The model under review builds one solid part; all positions refer to its coordinate system, in mm. A direction names the side the tool comes from. Coordinates: 2 decimals unless noted, no trailing zeros. Write each loop counter-clockwise with the first axis right and the second up, starting at its lowest first coordinate (ties: lowest second). Pieces come first, ordered by that corner, then holes. Notation, with made-up numbers: (70, -25.5) - (100, -25.5) arc R19 cw to (100, -10.5) - close; hole circle Ø4 at (60.25, 59). An arc over 180 degrees is marked (long way). Answer as CSV lines item,"result". Start each with the question number.
```python
from build123d import *

# Parameters (mm, degrees)
BOSS_EXTRUDE1_DEPTH = 8
CUT_EXTRUDE4_DEPTH  = 1.7
CUT_EXTRUDE5_DEPTH  = 7.4
CUT_EXTRUDE6_DEPTH  = 4.5
SKETCH3_R           = 2.2
CUT_EXTRUDE7_DEPTH  = 6
SKETCH1_10_R        = 1.6
CUT_EXTRUDE8_DEPTH  = 60.512855754


with BuildPart() as part:
    # Sketch1 → Boss-Extrude1 (new body)
    with BuildSketch(Plane.XY):
        with BuildLine():
            ThreePointArc((-32.17302157, 26.528978176), (-41.7, 0), (-32.17302157, -26.528978176))
            ThreePointArc((-32.17302157, -26.528978176), (-31.395541085, -31.395541085), (-26.528978176, -32.17302157))
            ThreePointArc((-26.528978176, -32.17302157), (0, -41.7), (26.528978176, -32.17302157))
            ThreePointArc((26.528978176, -32.17302157), (31.395541085, -31.395541085), (32.17302157, -26.528978176))
            ThreePointArc((32.17302157, -26.528978176), (41.7, 0), (32.17302157, 26.528978176))
            ThreePointArc((32.17302157, 26.528978176), (31.395541085, 31.395541085), (26.528978176, 32.17302157))
            ThreePointArc((26.528978176, 32.17302157), (0, 41.7), (-26.528978176, 32.17302157))
            ThreePointArc((-26.528978176, 32.17302157), (-31.395541085, 31.395541085), (-32.17302157, 26.528978176))
        make_face()
    extrude(amount=BOSS_EXTRUDE1_DEPTH)

    # Sketch1_7 → Cut-Extrude4 (cut)
    with BuildSketch(Plane.XY):
        with BuildLine():
            Line((-4.282842712, 9.374011537), (-9.475230868, 14.566399692))
            ThreePointArc((-9.475230868, 14.566399692), (-14.566399692, 14.566399692), (-14.566399692, 9.475230868))
            Line((-14.566399692, 9.475230868), (-9.374011537, 4.282842712))
            ThreePointArc((-9.374011537, 4.282842712), (-7.6, 0), (-9.374011537, -4.282842712))
            Line((-9.374011537, -4.282842712), (-14.566399692, -9.475230868))
            ThreePointArc((-14.566399692, -9.475230868), (-14.566399692, -14.566399692), (-9.475230868, -14.566399692))
            Line((-9.475230868, -14.566399692), (-4.282842712, -9.374011537))
            ThreePointArc((-4.282842712, -9.374011537), (0, -7.6), (4.282842712, -9.374011537))
            Line((4.282842712, -9.374011537), (9.475230868, -14.566399692))
            ThreePointArc((9.475230868, -14.566399692), (14.566399692, -14.566399692), (14.566399692, -9.475230868))
            Line((14.566399692, -9.475230868), (9.374011537, -4.282842712))
            ThreePointArc((9.374011537, -4.282842712), (7.6, 0), (9.374011537, 4.282842712))
            Line((9.374011537, 4.282842712), (14.566399692, 9.475230868))
            ThreePointArc((14.566399692, 9.475230868), (14.566399692, 14.566399692), (9.475230868, 14.566399692))
            Line((9.475230868, 14.566399692), (4.282842712, 9.374011537))
            ThreePointArc((4.282842712, 9.374011537), (0, 7.6), (-4.282842712, 9.374011537))
        make_face()
    extrude(amount=CUT_EXTRUDE4_DEPTH, mode=Mode.SUBTRACT)

    # Sketch1_8 → Cut-Extrude5 (cut)
    with BuildSketch(Plane.XY):
        Polygon((-7.1, -3.85), (7.1, -3.85), (7.1, 3.85), (7.1, 7.6), (-7.1, 7.6), (-7.1, 3.85), align=None)
    extrude(amount=CUT_EXTRUDE5_DEPTH, mode=Mode.SUBTRACT)

    # Sketch1_9 → Cut-Extrude6 (cut)
    with BuildSketch(Plane.XY):
        with BuildLine():
            Line((-4, 41.507710127), (-4, 9.10872459))
            ThreePointArc((-4, 9.10872459), (-2.137536533, 7.989719085), (2.1e-08, 7.6))
            ThreePointArc((2.1e-08, 7.6), (2.137536553, 7.989719093), (4, 9.10872459))
            Line((4, 9.10872459), (4, 41.507710127))
            ThreePointArc((4, 41.507710127), (0, 41.7), (-4, 41.507710127))
        make_face()
        with BuildLine():
            ThreePointArc((2.1e-08, 7.6), (-2.137536533, 7.989719085), (-4, 9.10872459))
            Line((-4, 9.10872459), (-4, 7.6))
            Line((-4, 7.6), (2.1e-08, 7.6))
        make_face()
        with BuildLine():
            ThreePointArc((4, 9.10872459), (2.137536553, 7.989719093), (2.1e-08, 7.6))
            Line((2.1e-08, 7.6), (4, 7.6))
            Line((4, 7.6), (4, 9.10872459))
        make_face()
    extrude(amount=CUT_EXTRUDE6_DEPTH, mode=Mode.SUBTRACT)

    # Sketch3 → Cut-Extrude7 (cut)
    with BuildSketch(Plane.XY.offset(8)):
        with Locations((-16, 0)):
            Circle(SKETCH3_R)
        with Locations(Location((16, 0, 0), (0, 0, 180))):
            Circle(SKETCH3_R)
        with Locations((0, -8)):
            Circle(SKETCH3_R)
    extrude(amount=-CUT_EXTRUDE7_DEPTH, mode=Mode.SUBTRACT)

    # Sketch1_10 → Cut-Extrude8 (cut, through all)
    with BuildSketch(Plane.XY):
        with Locations((-28.425692604, 28.425692604)):
            Circle(SKETCH1_10_R)
        with Locations((28.425692604, 28.425692604)):
            Circle(SKETCH1_10_R)
        with Locations((28.425692604, -28.425692604)):
            Circle(SKETCH1_10_R)
        with Locations((-28.425692604, -28.425692604)):
            Circle(SKETCH1_10_R)
    extrude(amount=CUT_EXTRUDE8_DEPTH, mode=Mode.SUBTRACT)


solid = part.part
```
(1) Add section D-D on x = 12. Give the boundary of the cut face in (y, z), then the cut area to 3 significant figures.
(2) Wall thickness on line 1 (X direction, y = 27, z = 7.5); line 2 (X direction, y = -1, z = 2.5); line 3 (Y direction, x = -29.5, z = 6): over which ranges is each line inside the solid? List them lowest first.
(3) For pin 1 (2 mm diameter, centred on x = -19, z = 5.5, fed in from -Y) (3 decimals); pin 2 (4 mm diameter, centred on y = 9.5, z = 3, fed in from +X); pin 3 (2 mm diameter, centred on x = 15.5, y = -0.5, fed in from +Z), all flat-tipped, find the tip position at first contact; note any pin that passes through.
(4) For faces 4 (the flat face through (16, 0, 2)), 5 (the flat face through (-6.92, -12.01, 0.84)), 6 (the flat face through (4, 24, 2)), list the 3-axis set-ups (+Z, -Z, +X, -X, +Y, -Y) from which the entire face can be reached by the end or side of a thin tool; tool diameter is ignored.
(5) Add section B-B on x = 0. Give the boundary of the cut face in (y, z), then the cut area to 3 significant figures.
(6) Add section C-C on z = 5.5. Give the number of separate pieces and of enclosed holes in the cut face, then the cut area to 3 significant figures.
(7) The part is to be moulded in two halves that separate along X. For faces 1 (the cylindrical face through (29.9, 27.8, 3.9)), 2 (the cylindrical face through (41.7, -0.4, 3.9)), 3 (the cylindrical face through (-41.7, 0.4, 3.9)), say which applies: released by +X, released by -X, zero draft, split by the parting line, or undercut.
(8) Add section A-A on y = 0. Give the boundary of the cut face in (x, z).
Reported:
1,outline,"(-39.94, 0) - (-15.62, 0) - (-15.62, 1.7) - (-6.91, 1.7) - (-6.91, 0) - (6.91, 0) - (6.91, 1.7) - (15.62, 1.7) - (15.62, 0) - (39.94, 0) - (39.94, 8) - (-39.94, 8) - close"
1,area,"609 mm²"
2,line 1,"-32.38 to -29.15, -27.7 to 27.7, 29.15 to 32.38"
2,line 2,"-41.69 to -17.96, -14.04 to -7.1, 7.1 to 14.04, 17.96 to 41.69"
2,line 3,"-32.49 to -29.61, -27.24 to 27.24, 29.61 to 32.49"
3,pin 1,"y = -37.615"
3,pin 2,"x = 41.02"
3,pin 3,"z = 2"
4,face 4,"+Z"
4,face 5,"-Z"
4,face 6,"-Z, +Y"
5,outline,"(-41.7, 0) - (-7.6, 0) - (-7.6, 1.7) - (-3.85, 1.7) - (-3.85, 7.4) - (7.6, 7.4) - (7.6, 4.5) - (41.7, 4.5) - (41.7, 8) - (-5.8, 8) - (-5.8, 2) - (-10.2, 2) - (-10.2, 8) - (-41.7, 8) - close"
5,area,"396 mm²"
6,separate pieces,"1"
6,enclosed holes,"8"
6,area,"5,290 mm²"
7,face 1,"undercut"
7,face 2,"released by +X"
7,face 3,"released by -X"
8,outline,"(-41.7, 0) - (-7.6, 0) - (-7.6, 1.7) - (-7.1, 1.7) - (-7.1, 7.4) - (7.1, 7.4) - (7.1, 1.7) - (7.6, 1.7) - (7.6, 0) - (41.7, 0) - (41.7, 8) - (18.2, 8) - (18.2, 2) - (13.8, 2) - (13.8, 8) - (-13.8, 8) - (-13.8, 2) - (-18.2, 2) - (-18.2, 8) - (-41.7, 8) - close"
